Verification items for the finished model (mm, model axes). A direction names the side the tool comes from. Coordinates: 2 decimals unless noted, no trailing zeros. Loops run counter-clockwise (first coordinate to the right, second up) from the corner with the lowest first, then second, coordinate; pieces in that order, holes last. Notation, with made-up numbers: (23.5, 5.25) - (28.5, 5.25) arc R13 cw to (28.5, 15.25) - close; hole circle Ø6 at (7.25, -39.75). An arc over 180 degrees is marked (long way). One line per item, written item: value. Start each with the question number.
(1) Set-up check for faces 1 (the face through (0, 32, 30)), 2 (the face through (-58.939, 40.231, 16.255)), 3 (the face through (30.75, 0.74, 17.85)): record each of +Z, -Z, +X, -X, +Y, -Y from which the full face is reachable in a straight line by a thin tool's end or side.
(2) Thickness scan on probe 1 along Z at (x, y) = (0, 17.5); probe 2 along X at (y, z) = (20.5, 27.5); probe 3 along Z at (x, y) = (-43.75, 43). Record the ranges inside material, lowest first. Write a range as [from, to].
(3) Section check A-A (x = -21.5). Record the boundary of the cut face in (y, z).
(4) Section check B-B (z = 6). Record the boundary of the cut face in (x, y).
(5) Section check C-C (y = 40). Record the boundary of the cut face in (x, z).
(6) Section check D-D (x = 27.45). Record the boundary of the cut face in (y, z).
(7) Gauge pin test, flat ends, axial feed: P1, Ø2.5, axis at x = -35.94, z = 32.35, coming from the +Y side; P2, Ø6, axis at y = 10, z = 17.5, coming from the -X side; P3, Ø7.5, axis at x = 26.5, z = 17.5, coming from the -Y side; P4, Ø2.5, axis at x = -39.95, z = 18, coming from the +Y side. Record the tip position at first contact, or that the pin passes through.
```python
from build123d import *

# Parameters (mm, degrees)
SKETCH1_W                 = 94.5
SKETCH1_H                 = 73
BOSS_EXTRUDE1_DEPTH       = 55
F_3_0MM_DOWEL_HOLE1_D     = 3
F_3_0MM_DOWEL_HOLE1_DEPTH = 30
F_3_0MM_DOWEL_HOLE1_TIP   = 0.901290929
SKETCH7_W                 = 60
SKETCH7_H                 = 31
CUT_EXTRUDE2_DEPTH        = 20
SHELL2_START              = 2
SHELL2_DEPTH              = 53
SHELL2_START_2            = 22
SHELL2_2_OUTLINE_W        = 64
SHELL2_2_OUTLINE_H        = 34
SHELL2_2_DEPTH            = 33
SHELL2_3_DEPTH            = 21.868454444
CUT_EXTRUDE3_DEPTH        = 1.5
F_3_0MM_DOWEL_HOLE3_D     = 3
SKETCH15_R                = 3.5
CUT_EXTRUDE4_DEPTH        = 3
SKETCH20_W                = 78.95760637
SKETCH20_H                = 8
BOSS_EXTRUDE2_DEPTH       = 10
SKETCH21_W                = 6
SKETCH21_H                = 6
BOSS_EXTRUDE3_DEPTH       = 30
F_3_0MM_DOWEL_HOLE5_D     = 3
F_3_0MM_DOWEL_HOLE5_DEPTH = 10
F_3_0MM_DOWEL_HOLE5_TIP   = 0.901290929
F_3_0MM_DOWEL_HOLE6_D     = 3
F_3_0MM_DOWEL_HOLE6_DEPTH = 10
F_3_0MM_DOWEL_HOLE6_TIP   = 0.901290929
SKETCH27_W                = 12
SKETCH27_H                = 6
CUT_EXTRUDE5_DEPTH        = 30
SKETCH28_R                = 6.5
BOSS_EXTRUDE4_DEPTH       = 25
FILLET1_R                 = 6
SKETCH29_R                = 5.25
CUT_EXTRUDE6_DEPTH        = 29


with BuildPart() as part:
    # Sketch1 → Boss-Extrude1 (new body)
    with BuildSketch(Plane(origin=(0, 0, 0), x_dir=(1, 0, 0), z_dir=(0, 1, 0))):
        Rectangle(SKETCH1_W, SKETCH1_H)
    extrude(amount=BOSS_EXTRUDE1_DEPTH)

    # Ø3.0mm Dowel Hole1
    with Locations(Plane(origin=(-43.75, 55, -33), x_dir=(0, 0, 1), z_dir=(0, 1, 0))):
        with Locations((0, 0), (0, 87.5), (66, 87.5), (66, 0)):
            Hole(F_3_0MM_DOWEL_HOLE1_D / 2, depth=F_3_0MM_DOWEL_HOLE1_DEPTH)
            with Locations((0, 0, -(F_3_0MM_DOWEL_HOLE1_DEPTH + F_3_0MM_DOWEL_HOLE1_TIP / 2))):  # 118° drill point
                Cone(0, F_3_0MM_DOWEL_HOLE1_D / 2, F_3_0MM_DOWEL_HOLE1_TIP, mode=Mode.SUBTRACT)

    # Sketch7 → Cut-Extrude2 (cut)
    with BuildSketch(Plane.XZ):
        with Locations((-6.25, 18)):
            Rectangle(SKETCH7_W, SKETCH7_H)
    extrude(amount=-CUT_EXTRUDE2_DEPTH, mode=Mode.SUBTRACT)

    # Shell2: read off the stored shape, not the designer's step
    # Shell2 outline → Shell2 (cut)
    with BuildSketch(Plane(origin=(0, 0, 0), x_dir=(1, 0, 0), z_dir=(0, 1, 0)).offset(SHELL2_START)):
        with BuildLine():
            Line((-45.25, 29.83772234), (-45.25, -29.83772234))
            ThreePointArc((-45.25, -29.83772234), (-41.275126266, -30.525126266), (-40.58772234, -34.5))
            Line((-40.58772234, -34.5), (-38.25, -34.5))
            Line((-38.25, -34.5), (-38.25, -0.5))
            Line((-38.25, -0.5), (25.75, -0.5))
            Line((25.75, -0.5), (25.75, -34.5))
            Line((25.75, -34.5), (40.58772234, -34.5))
            ThreePointArc((40.58772234, -34.5), (41.275126266, -30.525126266), (45.25, -29.83772234))
            Line((45.25, -29.83772234), (45.25, 29.83772234))
            ThreePointArc((45.25, 29.83772234), (41.275126266, 30.525126266), (40.58772234, 34.5))
            Line((40.58772234, 34.5), (-40.58772234, 34.5))
            ThreePointArc((-40.58772234, 34.5), (-41.275126266, 30.525126266), (-45.25, 29.83772234))
        make_face()
    extrude(amount=SHELL2_DEPTH, mode=Mode.SUBTRACT)

    # Shell2 2 outline → Shell2 2 (cut)
    with BuildSketch(Plane(origin=(0, 0, 0), x_dir=(1, 0, 0), z_dir=(0, 1, 0)).offset(SHELL2_START_2)):
        with Locations((-6.25, -17.5)):
            Rectangle(SHELL2_2_OUTLINE_W, SHELL2_2_OUTLINE_H)
    extrude(amount=SHELL2_2_DEPTH, mode=Mode.SUBTRACT)

    # Shell2 3 outline → Shell2 3 (cut)
    with BuildSketch(Plane(origin=(0, 0, 0), x_dir=(1, 0, 0), z_dir=(0, 1, 0)).offset(SHELL2_START)):
        with BuildLine():
            Line((-45.25, -29.83772234), (-45.25, -34.5))
            Line((-45.25, -34.5), (-40.58772234, -34.5))
            ThreePointArc((-40.58772234, -34.5), (-41.275126266, -30.525126266), (-45.25, -29.83772234))
        make_face()
        with BuildLine():
            Line((-45.25, 34.5), (-45.25, 29.83772234))
            ThreePointArc((-45.25, 29.83772234), (-41.275126266, 30.525126266), (-40.58772234, 34.5))
            Line((-40.58772234, 34.5), (-45.25, 34.5))
        make_face()
        with BuildLine():
            Line((45.25, 34.5), (40.58772234, 34.5))
            ThreePointArc((40.58772234, 34.5), (41.275126266, 30.525126266), (45.25, 29.83772234))
            Line((45.25, 29.83772234), (45.25, 34.5))
        make_face()
        with BuildLine():
            ThreePointArc((45.25, -29.83772234), (41.275126266, -30.525126266), (40.58772234, -34.5))
            Line((40.58772234, -34.5), (45.25, -34.5))
            Line((45.25, -34.5), (45.25, -29.83772234))
        make_face()
    extrude(amount=SHELL2_3_DEPTH, mode=Mode.SUBTRACT)

    # Shell2 4 outline → Shell2 4 (revolve)
    with BuildSketch(Plane(origin=(-43.75, 0, 33), x_dir=(1, 0, 0), z_dir=(0, 0, 1))):
        Polygon((0, 23.868454444), (0, 21.765442277), (3.5, 23.868454444), align=None)
    revolve(axis=Axis((-43.75, 0, 33), (0, 1, 0)))

    # Shell2 5 outline → Shell2 5 (revolve)
    with BuildSketch(Plane(origin=(43.75, 0, 33), x_dir=(1, 0, 0), z_dir=(0, 0, 1))):
        Polygon((0, 23.868454444), (0, 21.765442277), (3.5, 23.868454444), align=None)
    revolve(axis=Axis((43.75, 0, 33), (0, 1, 0)))

    # Shell2 6 outline → Shell2 6 (revolve)
    with BuildSketch(Plane(origin=(43.75, 0, -33), x_dir=(1, 0, 0), z_dir=(0, 0, 1))):
        Polygon((0, 23.868454444), (0, 21.765442277), (3.5, 23.868454444), align=None)
    revolve(axis=Axis((43.75, 0, -33), (0, 1, 0)))

    # Shell2 7 outline → Shell2 7 (revolve)
    with BuildSketch(Plane(origin=(-43.75, 0, -33), x_dir=(1, 0, 0), z_dir=(0, 0, 1))):
        Polygon((0, 23.868454444), (0, 21.765442277), (3.5, 23.868454444), align=None)
    revolve(axis=Axis((-43.75, 0, -33), (0, 1, 0)))

    # Sketch8 → Cut-Extrude3 (cut)
    with BuildSketch(Plane.XZ):
        with BuildLine():
            Line((23.75, 25), (23.75, 11))
            ThreePointArc((23.75, 11), (30.75, 18), (23.75, 25))
        make_face()
        with BuildLine():
            ThreePointArc((-36.25, 25), (-43.25, 18), (-36.25, 11))
            Line((-36.25, 11), (-36.25, 25))
        make_face()
    extrude(amount=-CUT_EXTRUDE3_DEPTH, mode=Mode.SUBTRACT)

    # Ø3.0mm Dowel Hole3 (through all)
    with Locations(Plane(origin=(27.45, 1.5, 18), x_dir=(0, 0, -1), z_dir=(0, -1, 0))):
        with Locations((0, 0), (0, -67.4)):
            Hole(F_3_0MM_DOWEL_HOLE3_D / 2)

    # Sketch15 → Cut-Extrude4 (cut)
    with BuildSketch(Plane.ZY.offset(-23.75)):
        with Locations((15.383017002, 11.670955046)):
            Circle(SKETCH15_R)
    extrude(amount=-CUT_EXTRUDE4_DEPTH, mode=Mode.SUBTRACT)

    # Sketch20 → Boss-Extrude2 (add)
    with BuildSketch(Plane(origin=(0, 22, 0), x_dir=(1, 0, 0), z_dir=(0, 1, 0))):
        with Locations((0.166869447, -30.5)):
            Rectangle(SKETCH20_W, SKETCH20_H)
    extrude(amount=BOSS_EXTRUDE2_DEPTH)

    # Sketch21 → Boss-Extrude3 (add)
    with BuildSketch(Plane(origin=(0, 2, 0), x_dir=(1, 0, 0), z_dir=(0, 1, 0))):
        with Locations((38.75, 26.5)):
            Rectangle(SKETCH21_W, SKETCH21_H)
    extrude(amount=BOSS_EXTRUDE3_DEPTH)

    # Ø3.0mm Dowel Hole5
    with Locations(Plane(origin=(0, 32, 0), x_dir=(1, 0, 0), z_dir=(0, 1, 0))):
        with Locations((36.25, -32), (-35.935310091, -32.352990413)):
            Hole(F_3_0MM_DOWEL_HOLE5_D / 2, depth=F_3_0MM_DOWEL_HOLE5_DEPTH)
            with Locations((0, 0, -(F_3_0MM_DOWEL_HOLE5_DEPTH + F_3_0MM_DOWEL_HOLE5_TIP / 2))):  # 118° drill point
                Cone(0, F_3_0MM_DOWEL_HOLE5_D / 2, F_3_0MM_DOWEL_HOLE5_TIP, mode=Mode.SUBTRACT)

    # Ø3.0mm Dowel Hole6
    with Locations(Plane(origin=(0, 32, 0), x_dir=(1, 0, 0), z_dir=(0, 1, 0))):
        with Locations((38.75, 26.5)):
            Hole(F_3_0MM_DOWEL_HOLE6_D / 2, depth=F_3_0MM_DOWEL_HOLE6_DEPTH)
            with Locations((0, 0, -(F_3_0MM_DOWEL_HOLE6_DEPTH + F_3_0MM_DOWEL_HOLE6_TIP / 2))):  # 118° drill point
                Cone(0, F_3_0MM_DOWEL_HOLE6_D / 2, F_3_0MM_DOWEL_HOLE6_TIP, mode=Mode.SUBTRACT)

    # Sketch27 → Cut-Extrude5 (cut)
    with BuildSketch(Plane(origin=(0, 0, -36.5), x_dir=(-1, 0, 0), z_dir=(0, 0, -1))):
        with Locations((26.25, 45)):
            Rectangle(SKETCH27_W, SKETCH27_H)
    extrude(amount=-CUT_EXTRUDE5_DEPTH, mode=Mode.SUBTRACT)

    # Sketch28 → Boss-Extrude4 (add)
    with BuildSketch(Plane.ZY.offset(47.25)):
        with Locations(Location((21.5, 40, 0), (0, 0, 180))):
            Circle(SKETCH28_R)
    extrude(amount=BOSS_EXTRUDE4_DEPTH)

    # Fillet1
    fillet1_edges = [part.edges().sort_by_distance(p)[0] for p in [
        (-47.25, 40, 28),
    ]]
    fillet(fillet1_edges, radius=FILLET1_R)

    # Sketch29 → Cut-Extrude6 (cut)
    with BuildSketch(Plane.ZY.offset(72.25)):
        with Locations((21.5, 40)):
            Circle(SKETCH29_R)
    extrude(amount=-CUT_EXTRUDE6_DEPTH, mode=Mode.SUBTRACT)


solid = part.part
```
Responses:
1. face 1: +Y
1. face 2: -X
1. face 3: -Y
2. probe 1: z = [-36.5, -34.5], [0.5, 2.5], [33.5, 36.5]
2. probe 2: x = [-47.25, -45.25], [-38.25, 25.75], [45.25, 47.25]
2. probe 3: z = [-36.5, -34.5], [-31.5, -29.5], [29.5, 31.5], [34.5, 36.5]
3. outline: (0, -36.5) - (42, -36.5) - (42, -34.5) - (2, -34.5) - (2, 0.5) - (22, 0.5) - (22, 26.5) - (32, 26.5) - (32, 34.5) - (55, 34.5) - (55, 36.5) - (0, 36.5) - (0, 33.5) - (20, 33.5) - (20, 2.5) - (0, 2.5) - close; (48, -36.5) - (55, -36.5) - (55, -34.5) - (48, -34.5) - close
4. outline: (-47.25, 0) - (-36.25, 0) - (-36.25, 20) - (23.75, 20) - (23.75, 0) - (47.25, 0) - (47.25, 55) - (45.25, 55) - (45.25, 2) - (25.75, 2) - (25.75, 22) - (-38.25, 22) - (-38.25, 2) - (-45.25, 2) - (-45.25, 55) - (-47.25, 55) - close
5. outline: (-72.25, 15) - (-53.25, 15) arc R6 cw to (-47.25, 9) - (-47.25, -36.5) - (47.25, -36.5) - (47.25, 36.5) - (-47.25, 36.5) - (-47.25, 34) arc R6 cw to (-53.25, 28) - (-72.25, 28) - (-72.25, 26.75) - (-45.25, 26.75) - (-45.25, 29.84) arc R3.5 ccw to (-40.59, 34.5) - (40.59, 34.5) arc R3.5 ccw to (45.25, 29.84) - (45.25, -29.84) arc R3.5 ccw to (40.59, -34.5) - (-40.59, -34.5) arc R3.5 ccw to (-45.25, -29.84) - (-45.25, 16.25) - (-72.25, 16.25) - close; hole circle Ø3 at (-43.75, -33); hole circle Ø3 at (-43.75, 33); hole circle Ø3 at (43.75, -33); hole circle Ø3 at (43.75, 33)
6. outline: (0, -36.5) - (55, -36.5) - (55, -34.5) - (2, -34.5) - (2, 16.5) - (1.5, 16.5) - (1.5, 12.06) - (0, 12.06) - close; (0, 23.94) - (1.5, 23.94) - (1.5, 19.5) - (2, 19.5) - (2, 34.5) - (22, 34.5) - (22, 26.5) - (32, 26.5) - (32, 34.5) - (55, 34.5) - (55, 36.5) - (0, 36.5) - close
7. P1: stops at y = 21.85
7. P2: stops at x = -47.25
7. P3: stops at y = 1.5
7. P4: passes through
